Here's the drawing with two shaded views (mm, measured from the low corner). I have some questions. A direction names the side the tool comes from. Give positions to 0.01 mm unless a question says otherwise; leave off trailing zeros. Loops run counter-clockwise (first coordinate to the right, second up) from the corner with the lowest first, then second, coordinate; pieces in that order, holes last. Notation, with made-up numbers: (79, 42) -> (112, 42) arc R23 ccw to (112, 61) -> close; hole circle Ø10 at (-31, 88.5). An arc over 180 degrees is marked (long way). Write each question's results on one line, items separated by ' | '. Start each with the question number.
Q1. If I drill on line 1 along Y through (x, z) = (55.5, 107); line 2 along Z through (x, y) = (79, 55); line 3 along Y through (x, z) = (109, 145), over which ranges is the centre line in solid material (lowest first)?
Q2. We'd pull the mould along Y, two halves only. Please class the marked faces 4, 5 and 6: released by +Y, released by -Y, zero draft, split by the parting line, or undercut.
Q3. If we section it at A-A, the plane z = 123: List the corners of the cut face in (x, y) for me.
Q4. If we section it at C-C, the plane z = 77: List the corners of the cut face in (x, y) for me.
Q5. If we section it at D-D, the plane y = 79: List the corners of the cut face in (x, z) for me, plus the area to 3 significant figures.
Q6. Will these pins go through, and if not, where does the flat tip stop? P1, Ø2, axis at x = 61, z = 143.5, coming from the +Y side; P2, Ø2, axis at y = 44.5, z = 106.5, coming from the -X side; P3, Ø6, axis at y = 37, z = 51, coming from the +X side.
Q7. Which directions (+Z, -Z, +X, -X, +Y, -Y) give clear straight access to the entire face, cutting with the end or side of a thin tool? Please do the marked faces 1, 2 and 3.
Q8. If we section it at B-B, the plane x = 41.5: List the corners of the cut face in (y, z) for me.
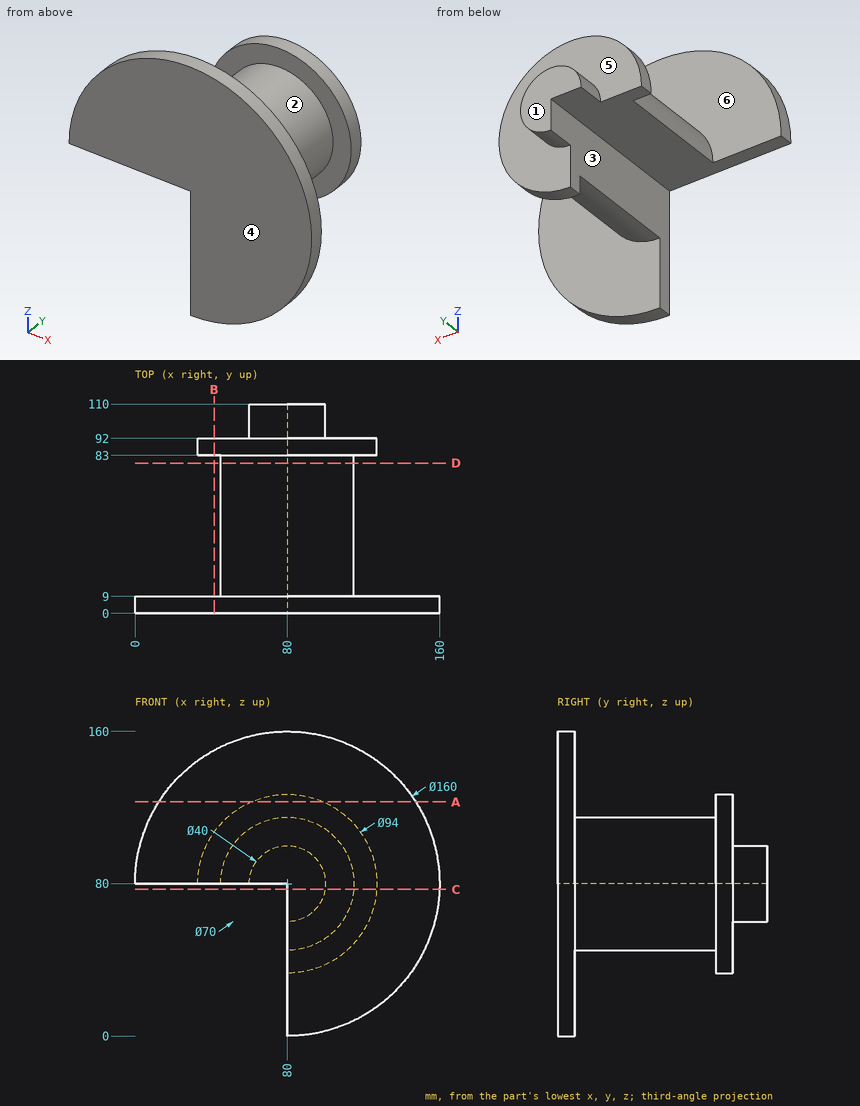
Final values:
1) line 1: y = 0 to 9, 83 to 92 | line 2: z = 80 to 114.99 | line 3: y = 0 to 9
2) face 4: released by -Y | face 5: released by +Y | face 6: undercut
3) outline: (12.54, 0) -> (147.46, 0) -> (147.46, 9) -> (12.54, 9) -> close; (61.03, 83) -> (98.97, 83) -> (98.97, 92) -> (61.03, 92) -> close
4) outline: (80, 0) -> (159.94, 0) -> (159.94, 9) -> (114.87, 9) -> (114.87, 83) -> (126.9, 83) -> (126.9, 92) -> (99.77, 92) -> (99.77, 110) -> (80, 110) -> close
5) outline: (45, 80) -> (80, 80) -> (80, 45) arc R35 ccw (long way) to start | area: 2,890 mm²
6) P1: stops at y = 9 | P2: stops at x = 56.03 | P3: stops at x = 103.43
7) face 1: +Z, -Z, +X, -X, +Y | face 2: none | face 3: -Z, -X, +Y, -Y
8) outline: (0, 80) -> (9, 80) -> (9, 150.13) -> (0, 150.13) -> close; (83, 80) -> (92, 80) -> (92, 106.96) -> (83, 106.96) -> close
